```python
from build123d import *

# Parameters (mm, degrees)
CHAMFER_1_SIZE      = 0.5
SKETCH_3_R          = 25
CUT_EXTRUDE_1_DEPTH = 12


with BuildPart() as part:
    # Эскиз1 → Повернуть1 (revolve)
    with BuildSketch(Plane.XY, mode=Mode.PRIVATE) as revolve_1_sk:
        with BuildLine():
            Line((0, 137), (-4, 137))
            Line((-4, 137), (-4, 32))
            Line((-4, 32), (-9.5, 32))
            Line((-9.5, 32), (-9.5, 20))
            Line((-9.5, 20), (-10.5, 20))
            ThreePointArc((-10.5, 20), (-18.901983424, 11.379145244), (-25, 1))
            Line((-25, 1), (-25, 0))
            Line((-25, 0), (0, 0))
            Line((0, 0), (0, 137))
        make_face()
    revolve(revolve_1_sk.sketch.rotate(Axis((0, 0, 0), (0, 1, 0)), 180), axis=Axis((0, 0, 0), (0, 1, 0)))  # turned: the seam where the file's is

    # Фаска1
    chamfer_1_edges = [part.edges().sort_by_distance(p)[0] for p in [
        (-4, 137, 0),
    ]]
    chamfer(chamfer_1_edges, length=CHAMFER_1_SIZE)

    # Эскиз3 → Вырез-Вытянуть1 (cut)
    with BuildSketch(Plane(origin=(0, 32, 0), x_dir=(1, 0, 0), z_dir=(0, 1, 0))):
        Circle(SKETCH_3_R)
        Polygon((0, 9.5), (-8.227241336, 4.75), (-8.227241336, -4.75), (0, -9.5), (8.227241336, -4.75), (8.227241336, 4.75), align=None, mode=Mode.SUBTRACT)
    extrude(amount=-CUT_EXTRUDE_1_DEPTH, mode=Mode.SUBTRACT)


solid = part.part
```
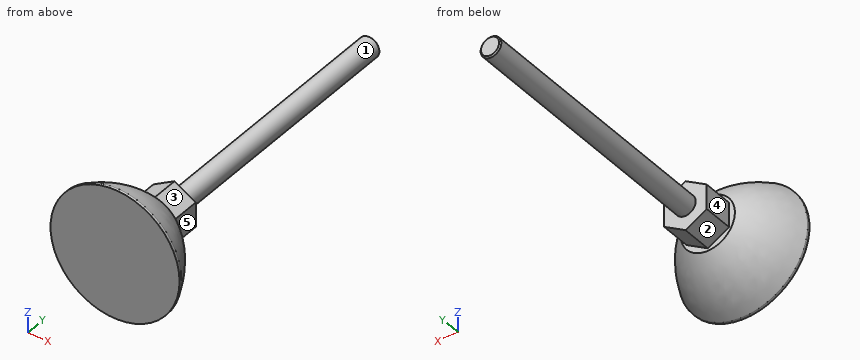
Can you work these out from the model? Positions are in its coordinate system, mm. Face numbers are marked on the shaded views. A direction names the side the tool comes from. Give positions to 0.01 mm unless a question says otherwise; leave off trailing zeros. Order: outer loops, then holes, each group sorted by start corner. A loop starts at its lowest first (then second) coordinate and runs counter-clockwise, first axis right, second up. Notation, with made-up numbers: M 56.5,42.5 L 71.5,42.5 A27 cw 71.5,58.5 Z; hole C 0,-40 d1. An arc over 180 degrees is marked long. One line per item, written item: value.
1) For P1, Ø6, axis at x = -5.5, y = 84.5, coming from the +Z side; P2, Ø5, axis at y = 25.5, z = 1, coming from the -X side; P3, Ø3, axis at y = 27.5, z = -0.5, coming from the +X side, each with a flat end and sliding along its axis, tell me the tip position at first contact or that it passes through.
Answer sheet:
P1: stops at z = 3.12
P2: stops at x = -8.23
P3: stops at x = 8.23
2) Please list where these lines run through material, in increasing order: line 1 along Y through (x, z) = (7, 6); line 2 along Y through (x, z) = (-2, 13); line 3 along X through (y, z) = (13.5, 4).
Answer sheet:
line 1: y = 0 to 20
line 2: y = 0 to 17.71
line 3: x = -16.72 to 16.72
3) I want a section at B-B, the plane y = 65. List the corners of the cut face in (x, z) for me.
Answer sheet:
outline: C 0,0 d8
4) On a 3-axis mill with a long thin cutter (end or side, diameter ignored), from which of +Z, -Z, +X, -X, +Y, -Y can I reach the whole of each face in a straight line? I mean the marked faces 1, 2, 3, 4 and 5. Say none if no direction works.
Answer sheet:
face 1: +Y
face 2: -Z, -X, +Y
face 3: +Z, +X, +Y
face 4: +Z, -Z, -X, +Y
face 5: +Z, -Z, +X, +Y
5) I want a section at A-A, the plane y = 28.5. List the corners of the cut face in (x, z) for me.
Answer sheet:
outline: M -8.23,-4.75 L 0,-9.5 L 8.23,-4.75 L 8.23,4.75 L 0,9.5 L -8.23,4.75 Z
